The model under review builds one solid part; all positions refer to its coordinate system, in mm. A direction names the side the tool comes from. Round coordinates to 2 decimals unless told otherwise and drop trailing zeros. Order: outer loops, then holes, each group sorted by start corner. A loop starts at its lowest first (then second) coordinate and runs counter-clockwise, first axis right, second up. Notation, with made-up numbers: M 41.5,-8.5 L 94.5,-8.5 A17 ccw 94.5,14.5 Z; hole C -24.5,15 d1. An arc over 180 degrees is marked long. One line per item, written item: value. Start each with the question number.
from build123d import *

# Parameters (mm, degrees)
SKETCH_1_R          = 5.2
SKETCH_1_R_2        = 2.5
EXTRUDE_1_DEPTH     = 3
EXTRUDE_START       = -2
SKETCH_3_R          = 5.2
SKETCH_3_R_2        = 2.5
EXTRUDE_3_DEPTH     = 2
SKETCH_7_R          = 2.5
CUT_EXTRUDE_1_DEPTH = 1
CUT_EXTRUDE_2_REACH = 53.662
SKETCH_9_R          = 2.5
CHAMFER_1_SIZE      = 1


with BuildPart() as part:
    # 스케치1 → 보스-돌출1 (new body)
    with BuildSketch(Plane.XY):
        Polygon((13.906175134, 23.803132686), (29.030703027, 23.803132686), (40.649680384, 12.184155329), (40.649680384, -28.196867314), (17.836321525, -28.196867314), (12.263074219, -23.196867314), (-3.200474103, -23.196867314), (-7.686189276, -28.196867314), (-43.049187557, -28.196867314), (-43.049187557, 8.903282862), (-28.149337734, 23.803132686), (-5.096572968, 23.803132686), (-0.180708362, 28.403132686), (8.990310529, 28.403132686), align=None)
        with Locations((22.449680384, -14.696867314)):
            Circle(SKETCH_1_R, mode=Mode.SUBTRACT)
        with Locations((-32.549187557, -3.196867314)):
            Circle(SKETCH_1_R, mode=Mode.SUBTRACT)
        with Locations((8.800246413, -2.196867314)):
            Circle(SKETCH_1_R_2, mode=Mode.SUBTRACT)
        with Locations((3.300246413, 22.303132686)):
            Circle(SKETCH_1_R_2, mode=Mode.SUBTRACT)
        with Locations((-21.199753587, 6.803132686)):
            Circle(SKETCH_1_R_2, mode=Mode.SUBTRACT)
    extrude(amount=EXTRUDE_1_DEPTH)

    # 스케치3 → 보스-돌출3 (add)
    # profile 1 of 2: a face of its own
    with BuildSketch(Plane.XY.offset(3).offset(EXTRUDE_START)):
        with Locations((-32.549187557, -3.196867314)):
            Circle(SKETCH_3_R)
        with Locations((-32.549187557, -3.196867314)):
            Circle(SKETCH_3_R_2, mode=Mode.SUBTRACT)
    # profile 2 of 2: a face of its own
    with BuildSketch(Plane.XY.offset(3).offset(EXTRUDE_START)):
        with Locations((22.449680384, -14.696867314)):
            Circle(SKETCH_3_R)
        with Locations((22.449680384, -14.696867314)):
            Circle(SKETCH_3_R_2, mode=Mode.SUBTRACT)
    extrude(amount=EXTRUDE_3_DEPTH)

    # 스케치7 → 컷-돌출1 (cut)
    with BuildSketch(Plane(origin=(0, 0, 0), x_dir=(-1, 0, 0), z_dir=(0, 0, -1))):
        with Locations((8.049187557, -24.196867314)):
            Circle(SKETCH_7_R)
        with Locations((6.149337734, 21.203132686)):
            Circle(SKETCH_7_R)
        with BuildLine():
            Line((-37.39408004, 7.870627017), (-37.39408004, 14.359426329))
            ThreePointArc((-37.39408004, 14.359426329), (-37.101186821, 15.066533111), (-36.39408004, 15.359426329))
            Line((-36.39408004, 15.359426329), (-33.149680384, 15.359426329))
            ThreePointArc((-33.149680384, 15.359426329), (-30.148436605, 14.116270452), (-28.905280727, 11.115026673))
            Line((-28.905280727, 11.115026673), (-28.905280727, 7.870627017))
            ThreePointArc((-28.905280727, 7.870627017), (-29.198173946, 7.163520236), (-29.905280727, 6.870627017))
            Line((-29.905280727, 6.870627017), (-36.39408004, 6.870627017))
            ThreePointArc((-36.39408004, 6.870627017), (-37.101186821, 7.163520236), (-37.39408004, 7.870627017))
        make_face()
    extrude(amount=-CUT_EXTRUDE_1_DEPTH, mode=Mode.SUBTRACT)

    # 스케치9 → 컷-돌출2 (cut, up to next)
    with BuildSketch(Plane(origin=(0, 0, 0), x_dir=(-1, 0, 0), z_dir=(0, 0, -1)), mode=Mode.PRIVATE) as cut_extrude_2_sk1:
        with Locations((-34.149680384, -13.196867314)):
            Circle(SKETCH_9_R)
    cut_extrude_2_tool1 = extrude(cut_extrude_2_sk1.sketch, amount=-CUT_EXTRUDE_2_REACH, mode=Mode.PRIVATE) & part.part
    # 스케치9 → 컷-돌출2 (cut, up to next)
    with BuildSketch(Plane(origin=(0, 0, 0), x_dir=(-1, 0, 0), z_dir=(0, 0, -1)), mode=Mode.PRIVATE) as cut_extrude_2_sk2:
        with Locations((-34.149680384, -23.196867314)):
            Circle(SKETCH_9_R)
    cut_extrude_2_tool2 = extrude(cut_extrude_2_sk2.sketch, amount=-CUT_EXTRUDE_2_REACH, mode=Mode.PRIVATE) & part.part
    # 스케치9 → 컷-돌출2 (cut, up to next)
    with BuildSketch(Plane(origin=(0, 0, 0), x_dir=(-1, 0, 0), z_dir=(0, 0, -1)), mode=Mode.PRIVATE) as cut_extrude_2_sk3:
        with Locations((36.549187557, -13.196867314)):
            Circle(SKETCH_9_R)
    cut_extrude_2_tool3 = extrude(cut_extrude_2_sk3.sketch, amount=-CUT_EXTRUDE_2_REACH, mode=Mode.PRIVATE) & part.part
    # 스케치9 → 컷-돌출2 (cut, up to next)
    with BuildSketch(Plane(origin=(0, 0, 0), x_dir=(-1, 0, 0), z_dir=(0, 0, -1)), mode=Mode.PRIVATE) as cut_extrude_2_sk4:
        with Locations((36.549187557, -23.196867314)):
            Circle(SKETCH_9_R)
    cut_extrude_2_tool4 = extrude(cut_extrude_2_sk4.sketch, amount=-CUT_EXTRUDE_2_REACH, mode=Mode.PRIVATE) & part.part
    add(cut_extrude_2_tool1.solids().sort_by_distance((34.14968, -13.196867, 0))[0], mode=Mode.SUBTRACT)
    add(cut_extrude_2_tool2.solids().sort_by_distance((34.14968, -23.196867, 0))[0], mode=Mode.SUBTRACT)
    add(cut_extrude_2_tool3.solids().sort_by_distance((-36.549188, -13.196867, 0))[0], mode=Mode.SUBTRACT)
    add(cut_extrude_2_tool4.solids().sort_by_distance((-36.549188, -23.196867, 0))[0], mode=Mode.SUBTRACT)

    # 모따기1
    chamfer_1_edges = [part.edges().sort_by_distance(p)[0] for p in [
        (40.649680384, -28.196867314, 1.5),
        (-43.049187557, -28.196867314, 1.5),
    ]]
    chamfer(chamfer_1_edges, length=CHAMFER_1_SIZE)


solid = part.part
Item 1: Consider section C-C, the plane x = -36.5. Give the boundary of the cut face in (y, z).
Item 2: Consider section A-A, the plane x = 21.5. Give the boundary of the cut face in (y, z).
Item 3: Clearance check with flat-ended pins moving along their axes: P1, Ø4.5, axis at x = 34.15, y = -13.2, coming from the -Z side; P2, Ø8, axis at x = -32.55, y = -3.2, coming from the +Z side; P3, Ø0.9, axis at x = 5, z = 1, coming from the -Y side; P4, Ø1.5, axis at x = -22, z = 1, coming from the +Y side. State where each tip first meets the part, or that it passes through.
Item 4: Consider section B-B, the plane z = 1.65. Count the separate pieces of the cut face and the enclosed holes in it, then the cut area to 3 significant figures.
Item 5: Wall thickness on L1, parallel to X at y = 9, z = 0.85; L2, parallel to X at y = -2, z = 1.3; L3, parallel to X at y = -12.5, z = 1.2: over which ranges is each line inside the solid? List them lowest first.
Item 6: Consider section D-D, the plane x = 34.5. Give the boundary of the cut face in (y, z).
Item 7: The part is to be moulded in two halves that separate along X. For faces 4 (the cylindrical face through (-38.934, -12.446, 1.479)), 5 (the flat face through (29, -28.197, 1)), 6 (the flat face through (-2.673, 26.071, 1.479)), say which applies: pulls with the +X half, pulls with the -X half, needs draft (parallel to the pull), parting line crosses it, or undercut.
Item 8: Machinability: for faces 1 (the cylindrical face through (6.303, -2.087, 1.479)), 2 (the flat face through (-5.41, -25.66, 1.48)), 3 (the cylindrical face through (21.322, -19.773, 0.493)), which of the approach directions +Z, -Z, +X, -X, +Y, -Y give a long, thin tool a straight path to every point of the face, cutting with its end or side? Answer none if there is none.
Computed:
1. outline: M -28.2,0 L -25.7,0 L -25.7,3 L -28.2,3 Z; M -20.7,0 L -15.7,0 L -15.7,3 L -20.7,3 Z; M -10.7,0 L -6.58,0 L -6.58,1 L 0.18,1 L 0.18,0 L 15.45,0 L 15.45,3 L -10.7,3 Z
2. outline: M -28.2,0 L -19.81,0 L -19.81,1 L -17.01,1 L -17.01,3 L -28.2,3 Z; M -12.38,1 L -9.58,1 L -9.58,0 L 23.8,0 L 23.8,3 L -12.38,3 Z
3. P1: passes through
3. P2: stops at z = 3
3. P3: stops at y = -23.2
3. P4: stops at y = 23.8
4. separate pieces: 1
4. enclosed holes: 9
4. area: 3,960 mm^2
5. L1: x = -42.95 to -22.39, -20.01 to 28.91, 37.39 to 40.65
5. L2: x = -43.05 to -34.74, -30.35 to 6.31, 11.29 to 40.65
5. L3: x = -43.05 to -38.95, -34.15 to 21.26, 23.64 to 31.75, 36.55 to 40.65
6. outline: M -28.2,0 L -25.67,0 L -25.67,3 L -28.2,3 Z; M -20.72,0 L -15.67,0 L -15.67,3 L -20.72,3 Z; M -10.72,0 L 6.87,0 L 6.87,1 L 15.36,1 L 15.36,0 L 18.33,0 L 18.33,3 L -10.72,3 Z
7. face 4: undercut
7. face 5: needs draft
7. face 6: pulls with the -X half
8. face 1: +Z, -Z
8. face 2: +Z, -Z, -Y
8. face 3: -Z
